Check sheet for the modelled part. Datum: model origin and axes. Units: mm. A direction names the side the tool comes from. Coordinates: 2 decimals unless noted, no trailing zeros. Order: outer loops, then holes, each group sorted by start corner. A loop starts at its lowest first (then second) coordinate and runs counter-clockwise, first axis right, second up.
from build123d import *

# Parameters (mm, degrees)
SKETCH1_W           = 30
SKETCH1_H           = 30
BOSS_EXTRUDE1_DEPTH = 30
CUT_EXTRUDE1_DEPTH  = 30
CUT_EXTRUDE2_DEPTH  = 30
CUT_EXTRUDE3_DEPTH  = 30
CUT_EXTRUDE4_DEPTH  = 30
CUT_EXTRUDE5_DEPTH  = 15
SKETCH6_R           = 1.5
CUT_EXTRUDE6_DEPTH  = 20
SKETCH8_R           = 1.5
CUT_EXTRUDE8_DEPTH  = 20
SKETCH10_R          = 1.5
CUT_EXTRUDE10_DEPTH = 20
CUT_EXTRUDE12_DEPTH = 52.961524227
SKETCH16_W          = 28.664479863
SKETCH16_H          = 34.476014612
CUT_EXTRUDE13_DEPTH = 7.5
SKETCH18_R          = 1
CUT_EXTRUDE14_DEPTH = 10
SKETCH19_R          = 1
CUT_EXTRUDE15_DEPTH = 10


with BuildPart() as part:
    # Sketch1 → Boss-Extrude1 (new body)
    with BuildSketch(Plane.XY):
        with Locations((15, 15)):
            Rectangle(SKETCH1_W, SKETCH1_H)
    extrude(amount=-BOSS_EXTRUDE1_DEPTH)

    # Sketch2 → Cut-Extrude1 (cut)
    with BuildSketch(Plane.XY):
        Polygon((15, 30), (30, 15), (45, 15), (45, 45.619084343), (15, 40.368332998), align=None)
    extrude(amount=-CUT_EXTRUDE1_DEPTH, mode=Mode.SUBTRACT)

    # Sketch3 → Cut-Extrude2 (cut)
    with BuildSketch(Plane.ZY):
        Polygon((0, 15), (-15, 30), (-15, 36.177250049), (9.539630377, 36.177250049), (9.539630377, 15), align=None)
    extrude(amount=-CUT_EXTRUDE2_DEPTH, mode=Mode.SUBTRACT)

    # Sketch4 → Cut-Extrude3 (cut)
    with BuildSketch(Plane.XZ):
        Polygon((15, 0), (30, -15), (40.227840819, -15), (40.227840819, 9.317096887), (15, 8.966367386), align=None)
    extrude(amount=-CUT_EXTRUDE3_DEPTH, mode=Mode.SUBTRACT)

    # 3DSketch1 → Cut-Extrude4 (cut)
    with BuildSketch(Plane(origin=(33.996909354, 3.570047518, -7.566956872), x_dir=(-0.34464530014522, 0.4926249601560642, 0.7990871452595439), z_dir=(-0.2113248654051872, 0.788675134594813, -0.5773502691896257))):
        Polygon((0, 0), (25.47550653, -16.637081723), (36.340550094, 0), (10.865043564, 16.637081723), align=None)
    extrude(amount=CUT_EXTRUDE4_DEPTH, mode=Mode.SUBTRACT)

    # Sketch5 → Cut-Extrude5 (cut)
    with BuildSketch(Plane(origin=(10, 10, 10), x_dir=(0.4082482904638628, 0.40824829046386263, -0.8164965809277264), z_dir=(0.5773502691896263, 0.5773502691896258, 0.5773502691896254))):
        Polygon((19.457058725, 2.946852636), (27.184465336, 5.017404997), (29.255017696, -2.710001614), (21.527611086, -4.780553975), align=None)
    extrude(amount=-CUT_EXTRUDE5_DEPTH, mode=Mode.SUBTRACT)

    # Sketch6 → Cut-Extrude6 (cut)
    with BuildSketch(Plane(origin=(0, 30, 0), x_dir=(1, 0, 0), z_dir=(0, 1, 0))):
        with Locations(Location((7.5, 22.5, 0), (0, 0, 270))):
            Circle(SKETCH6_R)
    extrude(amount=-CUT_EXTRUDE6_DEPTH, mode=Mode.SUBTRACT)

    # Sketch8 → Cut-Extrude8 (cut)
    with BuildSketch(Plane.XY):
        with Locations((7.5, 7.5)):
            Circle(SKETCH8_R)
    extrude(amount=-CUT_EXTRUDE8_DEPTH, mode=Mode.SUBTRACT)

    # Sketch10 → Cut-Extrude10 (cut)
    with BuildSketch(Plane(origin=(30, 0, 0), x_dir=(0, 0, -1), z_dir=(1, 0, 0))):
        with Locations(Location((22.5, 7.5, 0), (0, 0, 90))):
            Circle(SKETCH10_R)
    extrude(amount=-CUT_EXTRUDE10_DEPTH, mode=Mode.SUBTRACT)

    # Sketch14 → Cut-Extrude12 (cut, through all)
    with BuildSketch(Plane(origin=(0, 30, 0), x_dir=(1, 0, 0), z_dir=(0, 1, 0))):
        Polygon((0, 31.6), (32.521135015, 31.6), (32.521135015, 22.5), (6, 22.5), (0, 22.5), align=None)
    extrude(amount=-CUT_EXTRUDE12_DEPTH, mode=Mode.SUBTRACT)

    # Sketch16 → Cut-Extrude13 (cut)
    with BuildSketch(Plane.ZY):
        with Locations((-14.332239932, 17.238007306)):
            Rectangle(SKETCH16_W, SKETCH16_H)
    extrude(amount=-CUT_EXTRUDE13_DEPTH, mode=Mode.SUBTRACT)

    # Sketch18 → Cut-Extrude14 (cut)
    with BuildSketch(Plane.ZY.offset(-7.5)):
        with Locations(Location((-17.5, 24, 0), (0, 0, 270))):
            Circle(SKETCH18_R)
        with Locations(Location((-6, 3, 0), (0, 0, 270))):
            Circle(SKETCH18_R)
    extrude(amount=-CUT_EXTRUDE14_DEPTH, mode=Mode.SUBTRACT)

    # Sketch19 → Cut-Extrude15 (cut)
    with BuildSketch(Plane(origin=(0, 0, -22.5), x_dir=(-1, 0, 0), z_dir=(0, 0, -1))):
        with Locations((-25, 14)):
            Circle(SKETCH19_R)
        with Locations((-18, 3)):
            Circle(SKETCH19_R)
    extrude(amount=-CUT_EXTRUDE15_DEPTH, mode=Mode.SUBTRACT)


solid = part.part
(1) Thickness scan on probe 1 along Y at (x, z) = (18, -19.25); probe 2 along Y at (x, z) = (25.75, -21.5); probe 3 along Y at (x, z) = (22, -17.75). Record the ranges inside material, lowest first.
Filled in:
probe 1: y = 0 to 2, 4 to 13.99, 14.85 to 27
probe 2: y = 0 to 6.38, 8.62 to 13.34, 14.66 to 19.25
probe 3: y = 0 to 23
(2) Cross-section at D-D (x = 11). Enter the section's corners in (y, z), and give its area (3 significant figures).
Filled in:
outline: (0, -22.5) - (6, -22.5) arc R1.5 cw to (9, -22.5) - (30, -22.5) - (30, -15) - (15, 0) - (0, 0) - close; hole circle Ø2 at (3, -6); hole (8.58, -15.57) - (14.44, -21.42) - (18.1, -18.75) - (15.17, -10.75) - close; hole circle Ø2 at (24, -17.5)
area: 501 mm2
(3) Cross-section at A-A (y = 7.5). Enter the section's corners in (x, z), and give its area (3 significant figures).
Filled in:
outline: (7.5, -22.5) - (10, -22.5) - (10, -21) - (30, -21) - (30, -15) - (15, 0) - (9, 0) - (9, -20) - (7.5, -20) - close; hole (12.48, -15.96) - (13.78, -17.26) - (14.26, -15.49) - close
area: 332 mm2
(4) Tool access check on faces 4 (the flat face through (16.39, 18.1, -17.3)), 5 (the cylindrical face through (12, 3, -5)), 6 (the flat face through (8, 8, -20)), 7 (the flat face through (10, 7, -22)), 8 (the flat face through (25, 14, -12.5)). Record the directions out of +Z, -Z, +X, -X, +Y, -Y that give a thin tool (end or side, any length) a straight path to the whole face; none if there is none.
Filled in:
face 4: none
face 5: -X
face 6: +Z, -X
face 7: -Z, +X
face 8: -Z
(5) Release check for a two-part mould opening along X. For faces 1 (the flat face through (16, 0, -14)), 2 (the flat face through (18, 3, -12.5)), 3 (the flat face through (17.5, 24, -17)) record: +X half, -X half, draft (parallel to the pull), parting line (faces both ways), or undercut.
Filled in:
face 1: draft
face 2: undercut
face 3: -X half
(6) Go/stop test with flat-tipped pins: P1, Ø8, axis at y = 24.5, z = -13, coming from the +X side; P2, Ø1.6, axis at x = 8, y = 7.5, coming from the +Z side; P3, Ø6, axis at y = 6.5, z = -5, coming from the +X side. Record where each tip stops, or that it passes through.
Filled in:
P1: stops at x = 23.96
P2: stops at z = -20
P3: stops at x = 23
(7) Cross-section at C-C (z = -17.5). Enter the section's corners in (x, y), and give its area (3 significant figures).
Filled in:
outline: (7.5, 0) - (30, 0) - (30, 15) - (15, 30) - (7.5, 30) - (7.5, 25) - (17.5, 25) - (17.5, 23) - (7.5, 23) - (7.5, 9) arc R1.5 cw to (7.5, 6) - close; hole (7.99, 13.53) - (13.85, 7.67) - (20.25, 16.41) - (12.25, 19.34) - close; hole circle Ø2 at (18, 3); hole circle Ø2 at (25, 14)
area: 459 mm2
(8) Cross-section at B-B (x = 25). Enter the section's corners in (y, z), and give its area (3 significant figures).
Filled in:
outline: (0, -22.5) - (6, -22.5) arc R1.5 cw to (9, -22.5) - (13, -22.5) - (13, -12.5) - (15, -12.5) - (15, -22.5) - (20, -22.5) - (20, -15) - (15, -10) - (0, -10) - close
area: 214 mm2
